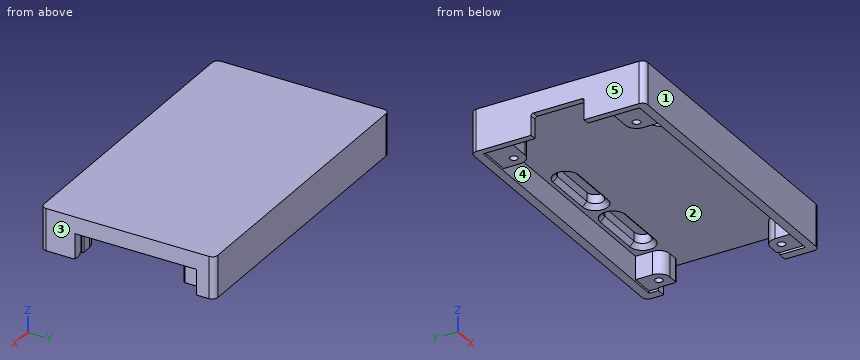
from build123d import *

# Parameters (mm, degrees)
SKETCH_1_R          = 2
SKETCH_1_R_2        = 0.7
EXTRUDE_5_DEPTH     = 3
EXTRUDE_6_DEPTH     = 7.6
SKETCH_1_8_R        = 2
SKETCH_1_8_R_2      = 0.7
EXTRUDE_7_DEPTH     = 7.2
SKETCH_1_9_W        = 1.2
SKETCH_1_9_H        = 9.6
EXTRUDE_8_DEPTH     = 3.7
FILLET_1_R          = 1
SKETCH_2_R          = 1.5
CUT_EXTRUDE_1_DEPTH = 2.4
CHAMFER_1_SIZE      = 0.8
FILLET_2_R          = 0.4
SKETCH_3_W          = 0.2
SKETCH_3_H          = 3.255284899
SKETCH_3_H_2        = 0.427
CUT_EXTRUDE_2_DEPTH = 4.2
FILLET_3_R          = 0.2


with BuildPart() as part:
    # Эскиз1 → Бобышка-Вытянуть5 (new body)
    with BuildSketch(Plane.XY):
        with BuildLine():
            Line((1.2, 20.5525), (1.2, 10.9525))
            Line((1.2, 10.9525), (1.2, 6.64))
            Line((1.2, 6.64), (5.383, 6.64))
            ThreePointArc((5.383, 6.64), (6.797213562, 6.054213562), (7.383, 4.64))
            Line((7.383, 4.64), (7.383, 1.6))
            Line((7.383, 1.6), (47.833, 1.6))
            Line((47.833, 1.6), (47.833, 4.64))
            ThreePointArc((47.833, 4.64), (48.418786438, 6.054213562), (49.833, 6.64))
            Line((49.833, 6.64), (51.984, 6.64))
            Line((51.984, 6.64), (51.984, 24.865))
            Line((51.984, 24.865), (49.833, 24.865))
            ThreePointArc((49.833, 24.865), (48.418786438, 25.450786438), (47.833, 26.865))
            Line((47.833, 26.865), (47.833, 29.905))
            Line((47.833, 29.905), (7.383, 29.905))
            Line((7.383, 29.905), (7.383, 26.865))
            ThreePointArc((7.383, 26.865), (6.797213562, 25.450786438), (5.383, 24.865))
            Line((5.383, 24.865), (1.2, 24.865))
            Line((1.2, 24.865), (1.2, 20.5525))
        make_face()
        Polygon((51.984, 6.213), (53.584, 6.213), (53.584, 28.213), (51.984, 28.213), (51.984, 24.865), (51.984, 6.64), align=None)
        with BuildLine():
            Line((51.984, 24.865), (51.984, 28.213))
            Line((51.984, 28.213), (51.984, 29.905))
            Line((51.984, 29.905), (47.833, 29.905))
            Line((47.833, 29.905), (47.833, 26.865))
            ThreePointArc((47.833, 26.865), (49.833, 28.865), (51.833, 26.865))
            ThreePointArc((51.833, 26.865), (51.247213562, 25.450786438), (49.833, 24.865))
            Line((49.833, 24.865), (51.984, 24.865))
        make_face()
        with Locations((49.833, 26.865)):
            Circle(SKETCH_1_R)
        with Locations((49.833, 26.865)):
            Circle(SKETCH_1_R_2, mode=Mode.SUBTRACT)
        with Locations((49.833, 26.865)):
            Circle(SKETCH_1_R_2)
        with BuildLine():
            Line((1.2, 29.905), (1.2, 24.865))
            Line((1.2, 24.865), (5.383, 24.865))
            ThreePointArc((5.383, 24.865), (3.968786438, 28.279213562), (7.383, 26.865))
            Line((7.383, 26.865), (7.383, 29.905))
            Line((7.383, 29.905), (1.2, 29.905))
        make_face()
        with Locations((5.383, 26.865)):
            Circle(SKETCH_1_R)
        with Locations((5.383, 26.865)):
            Circle(SKETCH_1_R_2, mode=Mode.SUBTRACT)
        with Locations((5.383, 26.865)):
            Circle(SKETCH_1_R_2)
        with BuildLine():
            Line((5.383, 6.64), (1.2, 6.64))
            Line((1.2, 6.64), (1.2, 1.6))
            Line((1.2, 1.6), (7.383, 1.6))
            Line((7.383, 1.6), (7.383, 4.64))
            ThreePointArc((7.383, 4.64), (3.968786438, 3.225786438), (5.383, 6.64))
        make_face()
        with Locations((5.383, 4.64)):
            Circle(SKETCH_1_R)
        with Locations((5.383, 4.64)):
            Circle(SKETCH_1_R_2, mode=Mode.SUBTRACT)
        with Locations((5.383, 4.64)):
            Circle(SKETCH_1_R_2)
        with BuildLine():
            Line((51.984, 1.6), (51.984, 6.213))
            Line((51.984, 6.213), (51.984, 6.64))
            Line((51.984, 6.64), (49.833, 6.64))
            ThreePointArc((49.833, 6.64), (51.247213562, 6.054213562), (51.833, 4.64))
            ThreePointArc((51.833, 4.64), (49.833, 2.64), (47.833, 4.64))
            Line((47.833, 4.64), (47.833, 1.6))
            Line((47.833, 1.6), (51.984, 1.6))
        make_face()
        with Locations((49.833, 4.64)):
            Circle(SKETCH_1_R)
        with Locations((49.833, 4.64)):
            Circle(SKETCH_1_R_2, mode=Mode.SUBTRACT)
        with Locations((49.833, 4.64)):
            Circle(SKETCH_1_R_2)
    extrude(amount=-EXTRUDE_5_DEPTH)

    # Эскиз1<7> → Бобышка-Вытянуть6 (add)
    with BuildSketch(Plane.XY):
        Polygon((0, 31.505), (0, 20.5525), (1.2, 20.5525), (1.2, 24.865), (1.2, 29.905), (7.383, 29.905), (47.833, 29.905), (51.984, 29.905), (51.984, 28.213), (53.584, 28.213), (53.584, 31.505), align=None)
        Polygon((0, 10.9525), (0, 0), (53.584, 0), (53.584, 6.213), (51.984, 6.213), (51.984, 1.6), (47.833, 1.6), (7.383, 1.6), (1.2, 1.6), (1.2, 6.64), (1.2, 10.9525), align=None)
    extrude(amount=-EXTRUDE_6_DEPTH)

    # Эскиз1<8> → Бобышка-Вытянуть7 (add)
    with BuildSketch(Plane.XY):
        with BuildLine():
            Line((51.984, 24.865), (51.984, 28.213))
            Line((51.984, 28.213), (51.984, 29.905))
            Line((51.984, 29.905), (47.833, 29.905))
            Line((47.833, 29.905), (47.833, 26.865))
            ThreePointArc((47.833, 26.865), (49.833, 28.865), (51.833, 26.865))
            ThreePointArc((51.833, 26.865), (51.247213562, 25.450786438), (49.833, 24.865))
            Line((49.833, 24.865), (51.984, 24.865))
        make_face()
        with Locations((49.833, 26.865)):
            Circle(SKETCH_1_8_R)
        with Locations((49.833, 26.865)):
            Circle(SKETCH_1_8_R_2, mode=Mode.SUBTRACT)
        with BuildLine():
            Line((1.2, 29.905), (1.2, 24.865))
            Line((1.2, 24.865), (5.383, 24.865))
            ThreePointArc((5.383, 24.865), (3.968786438, 28.279213562), (7.383, 26.865))
            Line((7.383, 26.865), (7.383, 29.905))
            Line((7.383, 29.905), (1.2, 29.905))
        make_face()
        with Locations((5.383, 26.865)):
            Circle(SKETCH_1_8_R)
        with Locations((5.383, 26.865)):
            Circle(SKETCH_1_8_R_2, mode=Mode.SUBTRACT)
        with BuildLine():
            Line((51.984, 1.6), (51.984, 6.213))
            Line((51.984, 6.213), (51.984, 6.64))
            Line((51.984, 6.64), (49.833, 6.64))
            ThreePointArc((49.833, 6.64), (51.247213562, 6.054213562), (51.833, 4.64))
            ThreePointArc((51.833, 4.64), (49.833, 2.64), (47.833, 4.64))
            Line((47.833, 4.64), (47.833, 1.6))
            Line((47.833, 1.6), (51.984, 1.6))
        make_face()
        with Locations((49.833, 4.64)):
            Circle(SKETCH_1_8_R)
        with Locations((49.833, 4.64)):
            Circle(SKETCH_1_8_R_2, mode=Mode.SUBTRACT)
        with BuildLine():
            Line((5.383, 6.64), (1.2, 6.64))
            Line((1.2, 6.64), (1.2, 1.6))
            Line((1.2, 1.6), (7.383, 1.6))
            Line((7.383, 1.6), (7.383, 4.64))
            ThreePointArc((7.383, 4.64), (3.968786438, 3.225786438), (5.383, 6.64))
        make_face()
        with Locations((5.383, 4.64)):
            Circle(SKETCH_1_8_R)
        with Locations((5.383, 4.64)):
            Circle(SKETCH_1_8_R_2, mode=Mode.SUBTRACT)
    extrude(amount=-EXTRUDE_7_DEPTH)

    # Эскиз1<9> → Бобышка-Вытянуть8 (add)
    with BuildSketch(Plane.XY):
        with Locations((0.6, 15.7525)):
            Rectangle(SKETCH_1_9_W, SKETCH_1_9_H)
    extrude(amount=-EXTRUDE_8_DEPTH)

    # Скругление1
    fillet_1_edges = [part.edges().sort_by_distance(p)[0] for p in [
        (0, 31.505, -3.8),
        (53.584, 31.505, -3.8),
        (53.584, 0, -3.8),
        (0, 0, -3.8),
    ]]
    fillet(fillet_1_edges, radius=FILLET_1_R)

    # Эскиз2 → Вырез-Вытянуть1 (cut)
    with BuildSketch(Plane(origin=(0, 0, -3), x_dir=(-1, 0, 0), z_dir=(0, 0, -1))):
        with Locations((-12.876, 4.513)):
            Circle(SKETCH_2_R)
        with BuildLine():
            Line((-44.808, 28.365), (-35.808, 28.365))
            ThreePointArc((-35.808, 28.365), (-34.308, 26.865), (-35.808, 25.365))
            Line((-35.808, 25.365), (-44.808, 25.365))
            ThreePointArc((-44.808, 25.365), (-46.308, 26.865), (-44.808, 28.365))
        make_face()
        with BuildLine():
            Line((-30.33, 28.365), (-21.33, 28.365))
            ThreePointArc((-21.33, 28.365), (-19.83, 26.865), (-21.33, 25.365))
            Line((-21.33, 25.365), (-30.33, 25.365))
            ThreePointArc((-30.33, 25.365), (-31.83, 26.865), (-30.33, 28.365))
        make_face()
    extrude(amount=-CUT_EXTRUDE_1_DEPTH, mode=Mode.SUBTRACT)

    # Фаска1
    chamfer_1_edges = [part.edges().sort_by_distance(p)[0] for p in [
        (46.308, 26.865, -3),
        (40.308, 25.365, -3),
        (34.308, 26.865, -3),
        (40.308, 28.365, -3),
        (31.83, 26.865, -3),
        (25.83, 25.365, -3),
        (19.83, 26.865, -3),
        (25.83, 28.365, -3),
        (14.376, 4.513, -3),
    ]]
    chamfer(chamfer_1_edges, length=CHAMFER_1_SIZE)

    # Скругление2
    fillet_2_edges = [part.edges().sort_by_distance(p)[0] for p in [
        (0.6, 20.5525, -3.7),
        (0.6, 10.9525, -3.7),
    ]]
    fillet(fillet_2_edges, radius=FILLET_2_R)

    # Эскиз3 → Вырез-Вытянуть2 (cut)
    with BuildSketch(Plane(origin=(0, 0, -7.2), x_dir=(-1, 0, 0), z_dir=(0, 0, -1))):
        with Locations((-51.884, 26.49264245)):
            Rectangle(SKETCH_3_W, SKETCH_3_H)
        with Locations((-51.884, 6.4265)):
            Rectangle(SKETCH_3_W, SKETCH_3_H_2)
    extrude(amount=-CUT_EXTRUDE_2_DEPTH, mode=Mode.SUBTRACT)

    # Скругление3
    fillet_3_edges = [part.edges().sort_by_distance(p)[0] for p in [
        (51.784, 24.865, -5.1),
        (51.784, 6.64, -5.1),
    ]]
    fillet(fillet_3_edges, radius=FILLET_3_R)


solid = part.part
For this review, take the finished solid that the model builds, in its own axes (mm). Face numbers are marked on the shaded views. A direction names the side the tool comes from. Round coordinates to 2 decimals unless told otherwise and drop trailing zeros. Loops run counter-clockwise (first coordinate to the right, second up) from the corner with the lowest first, then second, coordinate; pieces in that order, holes last. Notation, with made-up numbers: (58, 63.25) - (117, 63.25) arc R12 ccw to (117, 86.25) - close; hole circle Ø10 at (39.25, 24.5). An arc over 180 degrees is marked (long way). Answer as CSV lines item,"result".
(1) Consider section C-C on y = 13.5. Give the boundary of the cut face in (x, z), then the cut area to 3 significant figures.
Checked values:
outline,"(0, -3.7) - (1.2, -3.7) - (1.2, -3) - (53.58, -3) - (53.58, 0) - (0, 0) - close"
area,"162 mm2"
(2) Consider section D-D on x = 17.5. Give the boundary of the cut face in (y, z) (3 decimals), then the cut area to 3 significant figures.
Checked values:
outline,"(0, -7.6) - (1.6, -7.6) - (1.6, -3) - (29.905, -3) - (29.905, -7.6) - (31.505, -7.6) - (31.505, 0) - (0, 0) - close"
area,"109 mm2"
(3) Tool access review of the marked faces 4 and 5: name each direction out of +Z, -Z, +X, -X, +Y, -Y from which nothing blocks a thin tool from reaching the whole face with its end or side.
Checked values:
face 4,"-Z"
face 5,"+Z, -Z, -X, +Y, -Y"
(4) Mouldability with a two-part tool opening along Y and no side actions: class the marked faces 1, 2 and 3 as +Y half, -Y half, draft (parallel to the pull), parting line (faces both ways), or undercut.
Checked values:
face 1,"-Y half"
face 2,"undercut"
face 3,"draft"
(5) Consider section A-A on x = 40.5. Give the boundary of the cut face in (y, z) (3 decimals), then the cut area to 3 significant figures.
Checked values:
outline,"(0, -7.6) - (1.6, -7.6) - (1.6, -3) - (24.565, -3) - (25.365, -2.2) - (25.365, -0.6) - (28.365, -0.6) - (28.365, -2.2) - (29.165, -3) - (29.905, -3) - (29.905, -7.6) - (31.505, -7.6) - (31.505, 0) - (0, 0) - close"
area,"101 mm2"
(6) Wall thickness on line 1 (Y direction, x = 16.5, z = -4) (3 decimals); line 2 (X direction, y = 3.5, z = -5.5); line 3 (X direction, y = 26, z = -2): over which ranges is each line inside the solid? List them lowest first.
Checked values:
line 1,"y = 0 to 1.6, 29.905 to 31.505"
line 2,"x = 0 to 7.38, 47.83 to 53.58"
line 3,"x = 0 to 20.1, 31.56 to 34.58, 46.03 to 53.58"
(7) Consider section B-B on z = -1.25. Give the boundary of the cut face in (x, y) (3 decimals).
Checked values:
outline,"(0, 1) arc R1 ccw to (1, 0) - (52.584, 0) arc R1 ccw to (53.584, 1) - (53.584, 30.505) arc R1 ccw to (52.584, 31.505) - (1, 31.505) arc R1 ccw to (0, 30.505) - close; hole circle Ø3 at (12.876, 4.513); hole (21.33, 25.365) - (30.33, 25.365) arc R1.5 ccw to (30.33, 28.365) - (21.33, 28.365) arc R1.5 ccw to start; hole (35.808, 25.365) - (44.808, 25.365) arc R1.5 ccw to (44.808, 28.365) - (35.808, 28.365) arc R1.5 ccw to start"
(8) Insertion check: P1, Ø4.5, axis at x = 49.5, y = 27, coming from the -Z side; P2, Ø4, axis at x = 4.5, y = 28, coming from the -Z side; P3, Ø3.5, axis at y = 12, z = -5.5, coming from the +X side; P4, Ø5, axis at x = 24.5, y = 6, coming from the -Z side. Each pin has a flat end and moves straight along its axis. Give the tip position at first contact, or say it passes through.
Checked values:
P1,"stops at z = -7.2"
P2,"stops at z = -7.6"
P3,"stops at x = 1.2"
P4,"stops at z = -3"
